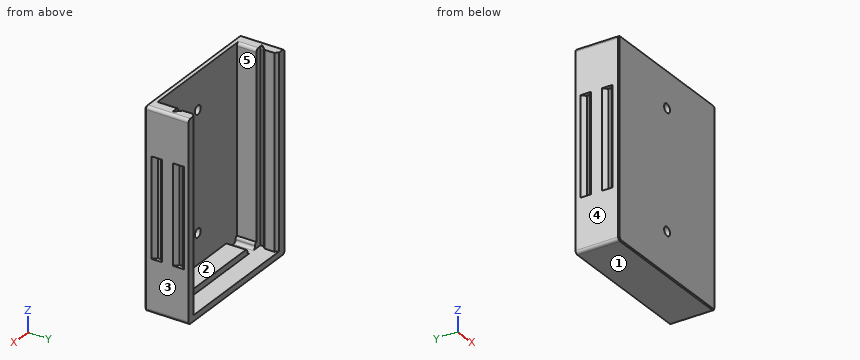
from build123d import *

# Parameters (mm, degrees)
SKETCH1_W           = 66.25
SKETCH1_H           = 97
BOSS_EXTRUDE1_DEPTH = 2.5
BOSS_EXTRUDE2_DEPTH = 97
SKETCH3_W           = 1
SKETCH3_H           = 3
BOSS_EXTRUDE3_DEPTH = 10
SKETCH4_W           = 74.25
SKETCH4_H           = 3
BOSS_EXTRUDE4_DEPTH = 22.12
SKETCH6_R           = 2.25
CUT_EXTRUDE1_DEPTH  = 67.448927945
FILLET1_R           = 1.5
CUT_EXTRUDE2_DEPTH  = 25
CHAMFER1_SIZE       = 0.5


with BuildPart() as part:
    # Sketch1 → Boss-Extrude1 (new body)
    with BuildSketch(Plane(origin=(0, 0, 0), x_dir=(1, 0, 0), z_dir=(0, 1, 0))):
        Rectangle(SKETCH1_W, SKETCH1_H)
    extrude(amount=BOSS_EXTRUDE1_DEPTH)

    # Sketch2 → Boss-Extrude2 (add)
    with BuildSketch(Plane.XY.offset(48.5)):
        Polygon((30.125, 2.5), (30.125, 12.5), (33.125, 12.5), (33.125, 14.12), (31.625, 15.62), (31.625, 20.62), (33.125, 22.12), (37.125, 22.12), (37.125, 0), (30.125, 0), align=None)
        Polygon((-31.625, 20.62), (-33.125, 22.12), (-37.125, 22.12), (-37.125, 0), (-30.125, 0), (-30.125, 2.5), (-30.125, 12.5), (-33.125, 12.5), (-33.125, 14.12), (-31.625, 15.62), align=None)
    extrude(amount=-BOSS_EXTRUDE2_DEPTH)

    # Sketch3 → Boss-Extrude3 (add)
    with BuildSketch(Plane(origin=(0, 2.5, 0), x_dir=(1, 0, 0), z_dir=(0, 1, 0))):
        Polygon((-23.125, 48.5), (-23.125, 45.5), (23.125, 45.5), (23.125, 48.5), (0, 48.5), align=None)
        with Locations((29.625, 47)):
            Rectangle(SKETCH3_W, SKETCH3_H)
        with Locations((-29.625, 47)):
            Rectangle(SKETCH3_W, SKETCH3_H)
    extrude(amount=BOSS_EXTRUDE3_DEPTH)

    # Sketch4 → Boss-Extrude4 (add)
    with BuildSketch(Plane.XZ):
        with Locations((0, -50)):
            Rectangle(SKETCH4_W, SKETCH4_H)
    extrude(amount=-BOSS_EXTRUDE4_DEPTH)

    # Sketch6 → Cut-Extrude1 (cut, through all)
    with BuildSketch(Plane(origin=(0, 2.5, 0), x_dir=(1, 0, 0), z_dir=(0, 1, 0))):
        with Locations(Location((0, 30, 0), (0, 0, 270))):
            Circle(SKETCH6_R)
        with Locations(Location((0, -30, 0), (0, 0, 270))):
            Circle(SKETCH6_R)
    extrude(amount=-CUT_EXTRUDE1_DEPTH, mode=Mode.SUBTRACT)

    # Fillet1
    # the kernel refuses this fillet: 1.5 mm, written as the material it adds along each edge
    with BuildSketch(Plane(origin=(29.125, 2.5, -48.5), x_dir=(-1, 0, 0), z_dir=(0, 1, 0)), Plane(origin=(-23.125, 2.5, -48.5), x_dir=(-1, 0, 0), z_dir=(0, 1, 0))) as fillet1_piece_1:
        with BuildLine():
            CenterArc((FILLET1_R, FILLET1_R), FILLET1_R, 180, 90)
            Line((0, FILLET1_R), (0, 0))
            Line((0, 0), (FILLET1_R, 0))
        make_face()
    extrude(amount=10)
    with BuildSketch(Plane(origin=(23.125, 2.5, -48.5), x_dir=(1, 0, 0), z_dir=(0, 1, 0)), Plane(origin=(-29.125, 2.5, -48.5), x_dir=(1, 0, 0), z_dir=(0, 1, 0))) as fillet1_piece_2:
        with BuildLine():
            CenterArc((FILLET1_R, -FILLET1_R), FILLET1_R, 90, 90)
            Line((0, -FILLET1_R), (0, 0))
            Line((0, 0), (FILLET1_R, 0))
        make_face()
    extrude(amount=10)
    # the kernel refuses this fillet: 1.5 mm, written as the material it takes off along each edge
    with BuildSketch(Plane(origin=(-33.125, 12.5, 48.5), x_dir=(-1, 0, 0), z_dir=(0, 1, 0))) as fillet1_2_piece_1_section:
        with BuildLine():
            CenterArc((FILLET1_R, -FILLET1_R), FILLET1_R, 90, 90)
            Line((0, -FILLET1_R), (0, 0))
            Line((0, 0), (FILLET1_R, 0))
        make_face()
    fillet1_2_piece_1 = extrude(amount=5.37, mode=Mode.PRIVATE)
    fillet1_2_piece_1 = split(fillet1_2_piece_1, bisect_by=Plane(origin=(-33.935, 13.31, 48.5), z_dir=(0.7071067811865467, -0.7071067811865483, 0)), keep=Keep.TOP, mode=Mode.PRIVATE)
    add(fillet1_2_piece_1, mode=Mode.SUBTRACT)
    with BuildSketch(Plane(origin=(33.125, 12.5, 48.5), x_dir=(1, 0, 0), z_dir=(0, 1, 0))) as fillet1_2_piece_2_section:
        with BuildLine():
            CenterArc((FILLET1_R, FILLET1_R), FILLET1_R, 180, 90)
            Line((0, FILLET1_R), (0, 0))
            Line((0, 0), (FILLET1_R, 0))
        make_face()
    fillet1_2_piece_2 = extrude(amount=5.37, mode=Mode.PRIVATE)
    fillet1_2_piece_2 = split(fillet1_2_piece_2, bisect_by=Plane(origin=(33.935, 13.31, 48.5), z_dir=(-0.7071067811865438, -0.7071067811865512, 0)), keep=Keep.TOP, mode=Mode.PRIVATE)
    add(fillet1_2_piece_2, mode=Mode.SUBTRACT)
    with BuildSketch(Plane(origin=(-30.125, 16.25, 48.5), x_dir=(-1, 0, 0), z_dir=(0, -1, 0)), Plane(origin=(30.125, 2.5, 48.5), x_dir=(1, 0, 0), z_dir=(0, 1, 0)), Plane(origin=(-23.125, 2.5, -45.5), x_dir=(1, 0, 0), z_dir=(0, 1, 0)), Plane(origin=(23.125, 2.5, -45.5), x_dir=(0, 0, -1), z_dir=(0, 1, 0))) as fillet1_2_piece_3:
        with BuildLine():
            CenterArc((FILLET1_R, FILLET1_R), FILLET1_R, 180, 90)
            Line((0, FILLET1_R), (0, 0))
            Line((0, 0), (FILLET1_R, 0))
        make_face()
    extrude(amount=13.75, mode=Mode.SUBTRACT)
    with BuildSketch(Plane(origin=(29.125, 2.5, -45.5), x_dir=(0, 0, -1), z_dir=(0, 1, 0))) as fillet1_2_piece_4:
        with BuildLine():
            CenterArc((1.414213562, -1.5), FILLET1_R, 90, 70.528779366)
            Line((0, -1), (0, 0))
            Line((0, 0), (1.414213562, 0))
        make_face()
    extrude(amount=13.535533906, mode=Mode.SUBTRACT)
    with BuildSketch(Plane(origin=(-29.125, 2.5, -45.5), x_dir=(0, 0, -1), z_dir=(0, 1, 0))) as fillet1_2_piece_5:
        with BuildLine():
            CenterArc((1.414213562, 1.5), FILLET1_R, 199.471220634, 70.528779366)
            Line((0, 1), (0, 0))
            Line((0, 0), (1.414213562, 0))
        make_face()
    extrude(amount=13.535533906, mode=Mode.SUBTRACT)
    with BuildSketch(Plane(origin=(37.125, 25.87, 48.5), x_dir=(-1, 0, 0), z_dir=(0, -1, 0)), Plane(origin=(-37.125, 25.87, 48.5), x_dir=(0, 0, -1), z_dir=(0, -1, 0)), Plane(origin=(-37.125, -3.75, -51.5), x_dir=(0, 0, 1), z_dir=(0, 1, 0))) as fillet1_2_piece_6:
        with BuildLine():
            CenterArc((FILLET1_R, FILLET1_R), FILLET1_R, 180, 90)
            Line((0, FILLET1_R), (0, 0))
            Line((0, 0), (FILLET1_R, 0))
        make_face()
    extrude(amount=29.62, mode=Mode.SUBTRACT)
    with BuildSketch(Plane(origin=(37.125, -3.75, -51.5), x_dir=(0, 0, 1), z_dir=(0, 1, 0))) as fillet1_2_piece_7:
        with BuildLine():
            CenterArc((FILLET1_R, -FILLET1_R), FILLET1_R, 90, 90)
            Line((0, -FILLET1_R), (0, 0))
            Line((0, 0), (FILLET1_R, 0))
        make_face()
    extrude(amount=29.62, mode=Mode.SUBTRACT)

    # Sketch7 → Cut-Extrude2 (cut, symmetric)
    with BuildSketch(Plane.XY):
        Polygon((-37.125, 8.75), (-35.125, 6.75), (-35.125, 5.25), (-37.125, 3.25), align=None)
        Polygon((-37.125, 19.75), (-35.125, 17.75), (-35.125, 16.25), (-37.125, 14.25), align=None)
        Polygon((37.125, 19.75), (37.125, 14.25), (35.125, 16.25), (35.125, 17.75), align=None)
        Polygon((37.125, 8.75), (37.125, 3.25), (35.125, 5.25), (35.125, 6.75), align=None)
    extrude(amount=CUT_EXTRUDE2_DEPTH, both=True, mode=Mode.SUBTRACT)

    # Chamfer1
    chamfer1_edges = [part.edges().sort_by_distance(p)[0] for p in [
        (0, 0, 48.5),
        (37.125, 0, -1.5),
        (-37.125, 0, -1.5),
        (0, 0, -51.5),
        (36.685660172, 0, -51.060660172),
        (-36.685660172, 0, -51.060660172),
        (-36.685660172, 0, 48.060660172),
        (36.685660172, 0, 48.060660172),
    ]]
    chamfer(chamfer1_edges, length=CHAMFER1_SIZE)


solid = part.part
Verification items for the finished model (mm, model axes). Face numbers are marked on the shaded views. A direction names the side the tool comes from. Give positions to 0.01 mm unless a question says otherwise; leave off trailing zeros. Write each loop counter-clockwise with the first axis right and the second up, starting at its lowest first coordinate (ties: lowest second). Pieces come first, ordered by that corner, then holes. Notation, with made-up numbers: M 66,1.25 L 72,1.25 A31 cw 72,34.25 Z; hole C 23,34.25 d6. An arc over 180 degrees is marked long. Use CSV: the item, a comma, the result in double quotes.
1) Cross-section at D-D (x = -18.5). Enter the section's corners in (y, z), plus the area to 3 significant figures.
Final values:
outline,"M 0,-51 L 0.5,-51.5 L 22.12,-51.5 L 22.12,-48.5 L 12.5,-48.5 L 12.5,-45.5 L 2.5,-45.5 L 2.5,48.5 L 0.5,48.5 L 0,48 Z"
area,"339 mm²"
2) Go/stop test with flat-tipped pins: pin 1 Ø0.8 at (y, z) = (17, 5.5) entering from +X (3 decimals); pin 2 Ø5 at (x, z) = (-27, -18.5) entering from +Y; pin 3 Ø2 at (x, y) = (36.5, 17.5) entering from +Z; pin 4 Ø1 at (x, y) = (36.5, 16.5) entering from -Z. Record where each tip stops, or that it passes through.
Final values:
pin 1,"x = 35.125"
pin 2,"y = 2.5"
pin 3,"z = 48.5"
pin 4,"z = -51.45"
3) Cross-section at C-C (y = 10). Enter the section's corners in (x, z) (3 decimals).
Final values:
outline,"M -37.125,-50 A1.5 ccw -35.625,-51.5 L 35.625,-51.5 A1.5 ccw 37.125,-50 L 37.125,47 A1.5 ccw 35.625,48.5 L 31.625,48.5 A1.5 ccw 30.125,47 L 30.125,-45.5 A1.5 ccw 29.125,-46.914 L 29.125,-47 A1.5 cw 27.625,-48.5 L 24.625,-48.5 A1.5 cw 23.125,-47 A1.5 ccw 21.625,-45.5 L -21.625,-45.5 A1.5 ccw -23.125,-47 A1.5 cw -24.625,-48.5 L -27.625,-48.5 A1.5 cw -29.125,-47 L -29.125,-46.914 A1.5 ccw -30.125,-45.5 L -30.125,47 A1.5 ccw -31.625,48.5 L -35.625,48.5 A1.5 ccw -37.125,47 Z"
4) Release check for a two-part mould opening along X. For the marked faces 3, 4 and 5 record: released by +X, released by -X, zero draft, split by the parting line, or undercut.
Final values:
face 3,"released by +X"
face 4,"released by -X"
face 5,"undercut"
5) Cross-section at B-B (x = 0). Enter the section's corners in (y, z), plus the area to 3 significant figures.
Final values:
outline,"M 0,-51 L 0.5,-51.5 L 22.12,-51.5 L 22.12,-48.5 L 12.5,-48.5 L 12.5,-45.5 L 2.5,-45.5 L 2.5,-32.25 L 0,-32.25 Z; M 0,-27.75 L 2.5,-27.75 L 2.5,27.75 L 0,27.75 Z; M 0,32.25 L 2.5,32.25 L 2.5,48.5 L 0.5,48.5 L 0,48 Z"
area,"316 mm²"
6) Material ranges on line 1 along X through (y, z) = (17.5, -44) (3 decimals); line 2 along X through (y, z) = (1.9, -30) (3 decimals); line 3 along Z through (x, y) = (3, 12.75), recorded low to high.
Final values:
line 1,"-37.125 to -31.625, 31.625 to 37.125"
line 2,"-37.125 to -2.25, 2.25 to 37.125"
line 3,"-51.5 to -48.5"
7) Access from +Z, -Z, +X, -X, +Y, -Y to the whole of each face (thin tool, end or side, straight path). Record for the marked faces 1 and 2.
Final values:
face 1,"-Z, +X, -X, +Y, -Y"
face 2,"+Z, +Y"
8) Cross-section at A-A (z = 30). Enter the section's corners in (x, y) (3 decimals), plus the area to 3 significant figures.
Final values:
outline,"M -37.125,0.5 L -36.625,0 L -2.25,0 L -2.25,2.5 L -30.125,2.5 L -30.125,12.5 L -33.125,12.5 L -33.125,14.12 L -31.625,15.62 L -31.625,20.62 L -33.125,22.12 L -37.125,22.12 Z; M 2.25,0 L 36.625,0 L 37.125,0.5 L 37.125,22.12 L 33.125,22.12 L 31.625,20.62 L 31.625,15.62 L 33.125,14.12 L 33.125,12.5 L 30.125,12.5 L 30.125,2.5 L 2.25,2.5 Z"
area,"411 mm²"
